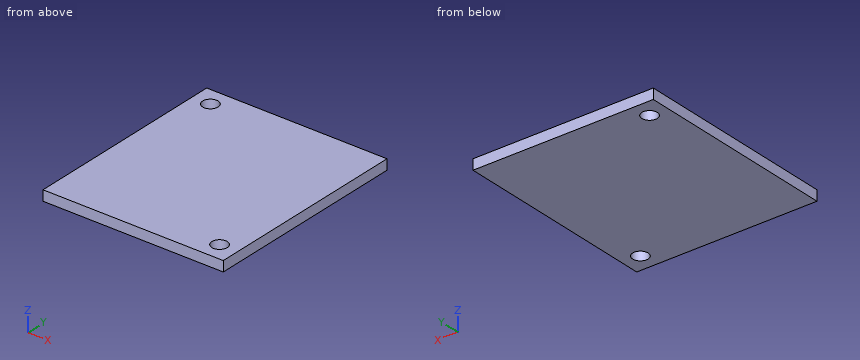
Autodesk Inventor part; units mm, degrees
ref_plane "YZ Plane" through (0, 0, 0) normal (1, 0, 0) x (0, 1, 0)
ref_plane "XZ Plane" through (0, 0, 0) normal (0, 1, 0) x (-1, 0, 0)
ref_plane "XY Plane" through (0, 0, 0) normal (0, 0, 1) x (1, 0, 0)
sketch "Sketch1" plane through (0, 0, 0) normal (0, 0, 1) x (1, 0, 0)
  line L0 (0, 0) -> (17.5, 0)
  line L1 (17.5, 0) -> (17.5, 20)
  line L2 (17.5, 20) -> (0, 20)
  line L3 (0, 20) -> (0, 0)
  line L4 (0, 0) -> (-17.5, 0)
  line L5 (-17.5, 0) -> (-17.5, -20)
  line L6 (-17.5, -20) -> (0, -20)
  line L7 (0, -20) -> (0, 0)
  line L8 (-17.5, -20) -> (17.5, -20)
  line L9 (17.5, -20) -> (17.5, 20)
  line L10 (17.5, 20) -> (-17.5, 20)
  line L11 (-17.5, 20) -> (-17.5, -20)
  point P0 (0, 20)
  point P1 (0, -20)
  dimension "d7" = 40
  dimension "d8" = 35
extrude "Extrusion1" add sketch "Sketch1" along normal blind 2
sketch "Sketch2" plane through (0, 0, 2) normal (0, 0, 1) x (1, 0, 0)
  line L0 (17.5, -20) -> (-17.5, -20) construction
  line L1 (17.5, 20) -> (17.5, -20) construction
  line L2 (-17.5, 20) -> (17.5, 20) construction
  line L3 (-17.5, -20) -> (-17.5, 20) construction
  line L4 (14, 16.5) -> (14, -16.5) construction
  line L5 (14, -16.5) -> (-14, -16.5) construction
  line L6 (-14, -16.5) -> (-14, 16.5) construction
  line L7 (-14, 16.5) -> (14, 16.5) construction
  circle A0 centre (-14, 16.5) radius 1.5
  circle A1 centre (14, -16.5) radius 1.5
  point P0 (0, 0)
  dimension "d9" = 3
  dimension "d10" = 3.5
extrude "Extrusion2" cut sketch "Sketch2" against normal through all
properties part number "Bottom"
Part model, mm, in its own coordinate system. Round coordinates to 2 decimals unless told otherwise and drop trailing zeros. Write each loop counter-clockwise with the first axis right and the second up, starting at its lowest first coordinate (ties: lowest second). Pieces come first, ordered by that corner, then holes. Notation, with made-up numbers: (-12.5, 47) -> (40.5, 47) arc R10 cw to (40.5, 53) -> close; hole circle Ø1 at (-33, 58). An arc over 180 degrees is marked (long way). Return JSON: item names as keys, results as strings. Group by question number.
Q1. Saw through at B-B on x = 14. Write the cut outline in (y, z), plus the area to 3 significant figures.
Q2. Probe L1, parallel to Y at x = -14, z = 0.55; L2, parallel to Y at x = 14, z = 0.95. List the from-to ranges inside material, lowest first. Write a range as [from, to].
Q3. Saw through at A-A on y = -16.5. Write the cut outline in (x, z).
Answer:
{
 "1": {"outline": "(-20, 0) -> (-18, 0) -> (-18, 2) -> (-20, 2) -> close; (-15, 0) -> (20, 0) -> (20, 2) -> (-15, 2) -> close", "area": "74.0 mm2"},
 "2": {"L1": "[-20, 15], [18, 20]", "L2": "[-20, -18], [-15, 20]"},
 "3": {"outline": "(-17.5, 0) -> (12.5, 0) -> (12.5, 2) -> (-17.5, 2) -> close; (15.5, 0) -> (17.5, 0) -> (17.5, 2) -> (15.5, 2) -> close"}
}
